For this review, take the finished solid that the model builds, in its own axes (mm). Face numbers are marked on the shaded views. Coordinates: 2 decimals unless noted, no trailing zeros. Order: outer loops, then holes, each group sorted by start corner. A loop starts at its lowest first (then second) coordinate and runs counter-clockwise, first axis right, second up.
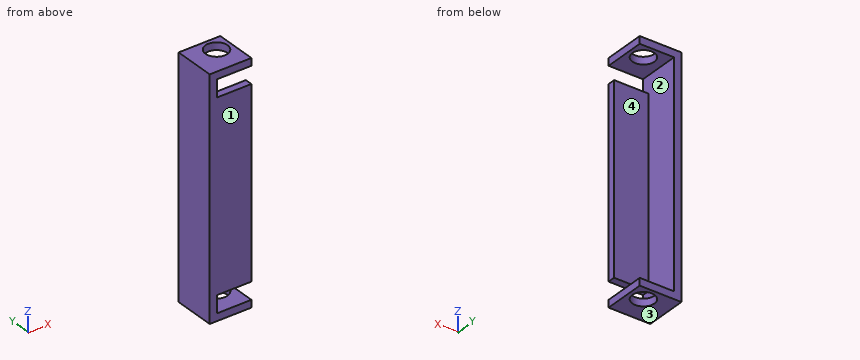
Autodesk Inventor part; units mm, degrees
ref_plane "YZ Plane" through (0, 0, 0) normal (1, 0, 0) x (0, 1, 0)
ref_plane "XZ Plane" through (0, 0, 0) normal (0, 1, 0) x (-1, 0, 0)
sketch "Sketch1" plane through (0, 0, 0) normal (0, 0, 1) x (1, 0, 0)
  circle A0 centre (0, 0) radius 2.25
  line L0 (-4, 3) -> (3, 3)
  line L1 (3, 3) -> (3, -4)
  line L2 (3, -4) -> (-4, -4)
  line L3 (-4, -4) -> (-4, 3)
  line L4 (-4, 3) -> (-5.5, 3)
  line L5 (-5.5, 3) -> (-5.5, -5.5)
  line L6 (-5.5, -5.5) -> (-4, -5.5)
  line L7 (-4, -5.5) -> (-4, 3)
  line L8 (3, -4) -> (-4, -4)
  line L9 (-4, -4) -> (-4, -5.5)
  line L10 (-4, -5.5) -> (3, -5.5)
  line L11 (3, -5.5) -> (3, -4)
  dimension "d0" = 4.5
  dimension "d1" = 4
  dimension "d2" = 4
  dimension "d3" = 3
  dimension "d5" = 3
  dimension "d6" = 1.5
  dimension "d7" = 1.5
extrude "Extrusion1" add sketch "Sketch1" along normal blind 1.5
extrude "Extrusion2" add sketch "Sketch1" along normal blind 46.5 contours L3 L7 L6 L5 L4 | L2 L11 L10 L7
ref_plane "Work Plane2" through (0, 0, 24) normal (0, 0, 1) x (1, 0, 0)
mirror "Mirror2" about plane through (0, 0, 24) normal (0, 0, 1) of "Extrusion1"
sketch "Sketch2" plane through (-4, -4, 1.5) normal (0, 1, 0) x (1, 0, 0)
  line L0 (7, 0) -> (7, -45)
  line L1 (0, 0) -> (7, 0)
  line L2 (7, 0) -> (7, -3.5)
  line L3 (7, -3.5) -> (0, -3.5)
  line L4 (0, -3.5) -> (0, 0)
  point P0 (4, 1.5)
  dimension "d13" = 3.5
extrude "Extrusion3" cut sketch "Sketch2" against normal blind 10
mirror "Mirror3" about plane through (0, 0, 24) normal (0, 0, 1) of "Extrusion3"
properties part number "Lifter"
1. Take a section at A-A, the plane x = 0. Give the boundary of the cut face in (y, z), plus the area to 3 significant figures.
Answer below:
outline: (-5.5, 0) - (-2.25, 0) - (-2.25, 1.5) - (-5.5, 1.5) - close; (-5.5, 5) - (-4, 5) - (-4, 43) - (-5.5, 43) - close; (-5.5, 46.5) - (-2.25, 46.5) - (-2.25, 48) - (-5.5, 48) - close; (2.25, 0) - (3, 0) - (3, 1.5) - (2.25, 1.5) - close; (2.25, 46.5) - (3, 46.5) - (3, 48) - (2.25, 48) - close
area: 69.0 mm2
2. Take a section at B-B, the plane y = 0. Give the boundary of the cut face in (x, z), plus the area to 3 significant figures.
Answer below:
outline: (-5.5, 0) - (-2.25, 0) - (-2.25, 1.5) - (-4, 1.5) - (-4, 46.5) - (-2.25, 46.5) - (-2.25, 48) - (-5.5, 48) - close; (2.25, 0) - (3, 0) - (3, 1.5) - (2.25, 1.5) - close; (2.25, 46.5) - (3, 46.5) - (3, 48) - (2.25, 48) - close
area: 79.5 mm2
3. To check wall thickness, follow L1, parallel to Z at x = -3.5, y = -5; L2, parallel to Z at x = 2.5, y = -0.25; L3, parallel to Y at x = 0, z = 47.5. State the ranges of each line that lie inside material, in increasing order.
Answer below:
L1: z = 0 to 1.5, 5 to 43, 46.5 to 48
L2: z = 0 to 1.5, 46.5 to 48
L3: y = -5.5 to -2.25, 2.25 to 3
4. Take a section at C-C, the plane z = 19. Give the boundary of the cut face in (x, y).
Answer below:
outline: (-5.5, -5.5) - (3, -5.5) - (3, -4) - (-4, -4) - (-4, 3) - (-5.5, 3) - close
5. The part is to be moulded in two halves that separate along Z. For the marked faces 1, 2, 3 and 4, say which applies: +Z half, -Z half, draft (parallel to the pull), parting line (faces both ways), or undercut.
Answer below:
face 1: draft
face 2: undercut
face 3: -Z half
face 4: undercut
6. Take a section at D-D, the plane y = -4.5. Give the boundary of the cut face in (x, z).
Answer below:
outline: (-5.5, 0) - (3, 0) - (3, 1.5) - (-4, 1.5) - (-4, 5) - (3, 5) - (3, 43) - (-4, 43) - (-4, 46.5) - (3, 46.5) - (3, 48) - (-5.5, 48) - close
